The listing builds one solid part. Answer for the finished solid, in the listing's coordinates (mm). A direction names the side the tool comes from. Coordinates: 2 decimals unless noted, no trailing zeros. Loops run counter-clockwise (first coordinate to the right, second up) from the corner with the lowest first, then second, coordinate; pieces in that order, holes last. Notation, with made-up numbers: (57, -21) - (70, -21) arc R25 ccw to (70, 3) - close; hole circle Ø7 at (53, 59). An arc over 180 degrees is marked (long way). Use one line per item in the form item = value. Start each with the question number.
```python
from build123d import *

# Parameters (mm, degrees)
SKETCH1_W           = 100
SKETCH1_H           = 26
SKETCH1_R           = 6.1
SKETCH1_R_2         = 4.1
BOSS_EXTRUDE1_DEPTH = 40
SKETCH2_W           = 100
SKETCH2_H           = 26
BOSS_EXTRUDE2_DEPTH = 29.4
CUT_EXTRUDE1_REACH  = 112.797
SKETCH3_W           = 58.5
SKETCH3_H           = 45
SKETCH4_R           = 2.6
CUT_EXTRUDE2_DEPTH  = 111.797111876
CUT_EXTRUDE3_DEPTH  = 4
SKETCH6_W           = 10
SKETCH6_H           = 18
CUT_EXTRUDE4_DEPTH  = 12.2
FILLET1_R           = 5


with BuildPart() as part:
    # Sketch1 → Boss-Extrude1 (new body)
    with BuildSketch(Plane.XY):
        with Locations((-50, 13)):
            Rectangle(SKETCH1_W, SKETCH1_H)
        with Locations((-90, 13)):
            Circle(SKETCH1_R, mode=Mode.SUBTRACT)
        with Locations((-66.5, 13)):
            Circle(SKETCH1_R_2, mode=Mode.SUBTRACT)
    boss_extrude1 = extrude(amount=BOSS_EXTRUDE1_DEPTH)

    # Sketch2 → Boss-Extrude2 (add)
    with BuildSketch(Plane(origin=(0, 0, 0), x_dir=(-1, 0, 0), z_dir=(0, 0, -1))):
        with Locations((50, 13)):
            Rectangle(SKETCH2_W, SKETCH2_H)
    boss_extrude2 = extrude(amount=BOSS_EXTRUDE2_DEPTH)

    # Sketch3 → Cut-Extrude1 (cut, up to next)
    with BuildSketch(Plane(origin=(0, 26, 0), x_dir=(1, 0, 0), z_dir=(0, 1, 0)), mode=Mode.PRIVATE) as cut_extrude1_sk1:
        with Locations((-29.25, -5.3)):
            Rectangle(SKETCH3_W, SKETCH3_H)
    cut_extrude1_tool1 = extrude(cut_extrude1_sk1.sketch, amount=-CUT_EXTRUDE1_REACH, mode=Mode.PRIVATE) & part.part
    cut_extrude1 = cut_extrude1_tool1.solids().sort_by_distance((-29.25, 26, 5.3))[0]
    add(cut_extrude1, mode=Mode.SUBTRACT)

    # Mirror2: Boss-Extrude1, Boss-Extrude2, Cut-Extrude1 across plane
    add(boss_extrude1.mirror(Plane(origin=(0, 0, 40), x_dir=(0, 0, 1), z_dir=(-1, 0, 0))))
    add(boss_extrude2.mirror(Plane(origin=(0, 0, 40), x_dir=(0, 0, 1), z_dir=(-1, 0, 0))))
    add(cut_extrude1.mirror(Plane(origin=(0, 0, 40), x_dir=(0, 0, 1), z_dir=(-1, 0, 0))), mode=Mode.SUBTRACT)

    # Sketch4 → Cut-Extrude2 (cut, through all)
    with BuildSketch(Plane(origin=(0, 26, 0), x_dir=(1, 0, 0), z_dir=(0, 1, 0))):
        with Locations(Location((3.5, 23.3, 0), (0, 0, 180))):
            Circle(SKETCH4_R)
        with Locations(Location((29.5, 23.3, 0), (0, 0, 180))):
            Circle(SKETCH4_R)
    cut_extrude2 = extrude(amount=-CUT_EXTRUDE2_DEPTH, mode=Mode.SUBTRACT)

    # Sketch5 → Cut-Extrude3 (cut)
    with BuildSketch(Plane.XZ):
        Polygon((34.234272207, -23.3), (31.867136104, -19.2), (27.132863896, -19.2), (24.765727793, -23.3), (27.132863896, -27.4), (31.867136104, -27.4), align=None)
        Polygon((-1.234272207, -23.3), (1.132863896, -27.4), (5.867136104, -27.4), (8.234272207, -23.3), (5.867136104, -19.2), (1.132863896, -19.2), align=None)
    cut_extrude3 = extrude(amount=-CUT_EXTRUDE3_DEPTH, mode=Mode.SUBTRACT)

    # Mirror3: Cut-Extrude2, Cut-Extrude3 across plane
    add(cut_extrude2.mirror(Plane.XY.offset(5.3)), mode=Mode.SUBTRACT)
    add(cut_extrude3.mirror(Plane.XY.offset(5.3)), mode=Mode.SUBTRACT)

    # Sketch6 → Cut-Extrude4 (cut)
    with BuildSketch(Plane.XY.offset(40)):
        with Locations((-23.2, 13)):
            Rectangle(SKETCH6_W, SKETCH6_H)
    extrude(amount=-CUT_EXTRUDE4_DEPTH, mode=Mode.SUBTRACT)

    # Fillet1
    fillet1_edges = [part.edges().sort_by_distance(p)[0] for p in [
        (-58.5, 26, 5.3),
        (-58.5, 0, 5.3),
        (100, 0, 5.3),
        (100, 26, 5.3),
        (-100, 0, 5.3),
        (-100, 26, 5.3),
        (58.5, 0, 5.3),
        (58.5, 26, 5.3),
    ]]
    fillet(fillet1_edges, radius=FILLET1_R)


solid = part.part
```
(1) For faces 1 (the face through (7.034, 1.972, 35.979)), 2 (the face through (-66, 13, 0)), 3 (the face through (60, 24.57, 4.98)), determine the directions among +Z, -Z, +X, -X, +Y, -Y from which every point of the face is accessible in a straight line to the end or side of a thin tool.
(2) Find the intervals of material crossed by probe 1 along Z at (x, y) = (29.5, 17.5); probe 2 along Z at (x, y) = (22, 20.75); probe 3 along X at (y, z) = (10, 16), in increasing order. Write a range as from..to.
(3) Each of these flat-tipped pins is pushed along its axis until it touches: pin 1 Ø2 at (y, z) = (23, 10) entering from +X; pin 2 Ø12 at (x, z) = (-3.5, -7.5) entering from -Y; pin 3 Ø7 at (x, z) = (3.5, -23.3) entering from -Y. Where does it stop, or does it pass through?
(4) A cutting plane is placed at C-C (z = -12). Determine the outline of the cut face in (x, y), then the cut area to 3 significant figures.
(5) A cutting plane is placed at A-A (z = 18). Determine the outline of the cut face in (x, y).
(6) A cutting plane is placed at D-D (x = 66.5). Determine the outline of the cut face in (y, z), then the cut area to 3 significant figures.
(7) Determine the mould class of faces 4 (the face through (-1, 13, -29.4)), 5 (the face through (6, 4, -21)), 6 (the face through (98, 25, 5)), 7 (the face through (-0.034, 1.972, -21.221)) for opening direction X: +X half, -X half, draft (parallel to the pull), parting line (faces both ways), or undercut.
(8) A cutting plane is placed at B-B (x = 3.5). Determine the outline of the cut face in (y, z), then the cut area to 3 significant figures.
Evaluation:
q1.face_1 = -Y
q1.face_2 = +Z
q1.face_3 = +Y
q2.probe_1 = -29.4..-25.9, -20.7..-17.2, 27.8..31.3, 36.5..40
q2.probe_2 = -29.4..-17.2, 27.8..40
q2.probe_3 = -100..-95.31, -84.69..-69.29, -63.71..-58.5, 58.5..63.71, 69.29..84.69, 95.31..100
q3.pin_1 = 99.9
q3.pin_2 = through
q3.pin_3 = 4
q4.outline = (-100, 5) arc R5 ccw to (-95, 0) - (-63.5, 0) arc R5 ccw to (-58.5, 5) - (-58.5, 21) arc R5 ccw to (-63.5, 26) - (-95, 26) arc R5 ccw to (-100, 21) - close; (58.5, 5) arc R5 ccw to (63.5, 0) - (95, 0) arc R5 ccw to (100, 5) - (100, 21) arc R5 ccw to (95, 26) - (63.5, 26) arc R5 ccw to (58.5, 21) - close
q4.area = 2,120 mm^2
q5.outline = (-100, 5) arc R5 ccw to (-95, 0) - (-63.5, 0) arc R5 ccw to (-58.5, 5) - (-58.5, 21) arc R5 ccw to (-63.5, 26) - (-95, 26) arc R5 ccw to (-100, 21) - close; (58.5, 5) arc R5 ccw to (63.5, 0) - (95, 0) arc R5 ccw to (100, 5) - (100, 21) arc R5 ccw to (95, 26) - (63.5, 26) arc R5 ccw to (58.5, 21) - close; hole circle Ø12.2 at (-90, 13); hole circle Ø8.2 at (-66.5, 13); hole circle Ø8.2 at (66.5, 13); hole circle Ø12.2 at (90, 13)
q6.outline = (0, -29.4) - (26, -29.4) - (26, 40) - (17.1, 40) - (17.1, 0) - (8.9, 0) - (8.9, 40) - (0, 40) - close
q6.area = 1,480 mm^2
q7.face_4 = draft
q7.face_5 = undercut
q7.face_6 = +X half
q7.face_7 = undercut
q8.outline = (0, -29.4) - (26, -29.4) - (26, -25.9) - (4, -25.9) - (4, -27.4) - (0, -27.4) - close; (0, -19.2) - (4, -19.2) - (4, -20.7) - (26, -20.7) - (26, -17.2) - (0, -17.2) - close; (0, 27.8) - (26, 27.8) - (26, 31.3) - (4, 31.3) - (4, 29.8) - (0, 29.8) - close; (0, 38) - (4, 38) - (4, 36.5) - (26, 36.5) - (26, 40) - (0, 40) - close
q8.area = 340 mm^2
